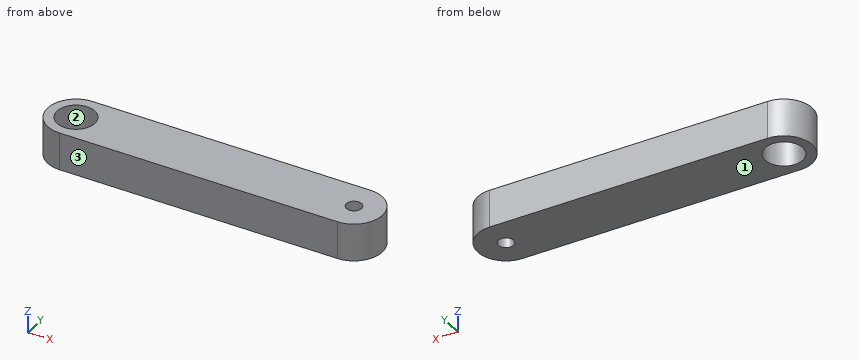
```python
from build123d import *

# Parameters (mm, degrees)
BOSS_EXTRU_1_DEPTH      = 10
ESQUISSE2_R             = 5
ESQUISSE2_R_2           = 2
ENL_V_MAT_EXTRU_1_DEPTH = 82.464716289


with BuildPart() as part:
    # Esquisse1 → Boss.-Extru.1 (new body)
    with BuildSketch(Plane.XY):
        with BuildLine():
            Line((0, -7.5), (-73, -7.5))
            ThreePointArc((-73, -7.5), (-80.5, 0), (-73, 7.5))
            Line((-73, 7.5), (0, 7.5))
            ThreePointArc((0, 7.5), (7.5, 0), (0, -7.5))
        make_face()
    extrude(amount=BOSS_EXTRU_1_DEPTH)

    # Esquisse2 → Enlèv. mat.-Extru.1 (cut, through all)
    with BuildSketch(Plane.XY.offset(10)):
        with Locations((-73, 0)):
            Circle(ESQUISSE2_R)
        Circle(ESQUISSE2_R_2)
    extrude(amount=-ENL_V_MAT_EXTRU_1_DEPTH, mode=Mode.SUBTRACT)


solid = part.part
```
The listing builds one solid part. Answer for the finished solid, in the listing's coordinates (mm). Face numbers are marked on the shaded views. Coordinates: 2 decimals unless noted, no trailing zeros. Write each loop counter-clockwise with the first axis right and the second up, starting at its lowest first coordinate (ties: lowest second). Pieces come first, ordered by that corner, then holes. Notation, with made-up numbers: (-17, 69) - (-6, 69) arc R14 ccw to (-6, 95) - close; hole circle Ø11 at (-35.5, -23.75). An arc over 180 degrees is marked (long way). Return JSON: item names as keys, results as strings. Group by question number.
Q1. The part is cut by section A-A on y = 0. Write down the section's boundary in (x, z), and give its area (3 significant figures).
Q2. For a pull along Y with two mould halves and no side action, classify the marked faces 1, 2 and 3 as +Y half, -Y half, draft (parallel to the pull), parting line (faces both ways), or undercut.
Q3. Find the intervals of material crossed by line 1 along Y through (x, z) = (-73, 6.25); line 2 along X through (y, z) = (1.5, 9.25); line 3 along X through (y, z) = (-1, 8), in increasing order. Write a range as [from, to].
Q4. A flat-ended cylindrical pin translates along its axis: pin 1 Ø6 at (y, z) = (3.5, 3) entering from -X. Find the tip coordinate at first contact, or state that the pin passes through.
Q5. The part is cut by section B-B on z = 2.75. Write down the section's boundary in (x, y), and give its area (3 significant figures).
Evaluation:
{
 "1": {"outline": "(-80.5, 0) - (-78, 0) - (-78, 10) - (-80.5, 10) - close; (-68, 0) - (-2, 0) - (-2, 10) - (-68, 10) - close; (2, 0) - (7.5, 0) - (7.5, 10) - (2, 10) - close", "area": "740 mm2"},
 "2": {"face 1": "draft", "face 2": "undercut", "face 3": "-Y half"},
 "3": {"line 1": "y = [-7.5, -5], [5, 7.5]", "line 2": "x = [-80.35, -77.77], [-68.23, -1.32], [1.32, 7.35]", "line 3": "x = [-80.43, -77.9], [-68.1, -1.73], [1.73, 7.43]"},
 "4": {"pin 1": "stops at x = -80.48"},
 "5": {"outline": "(-73, -7.5) - (0, -7.5) arc R7.5 ccw to (0, 7.5) - (-73, 7.5) arc R7.5 ccw to start; hole circle Ø10 at (-73, 0); hole circle Ø4 at (0, 0)", "area": "1,180 mm2"}
}
